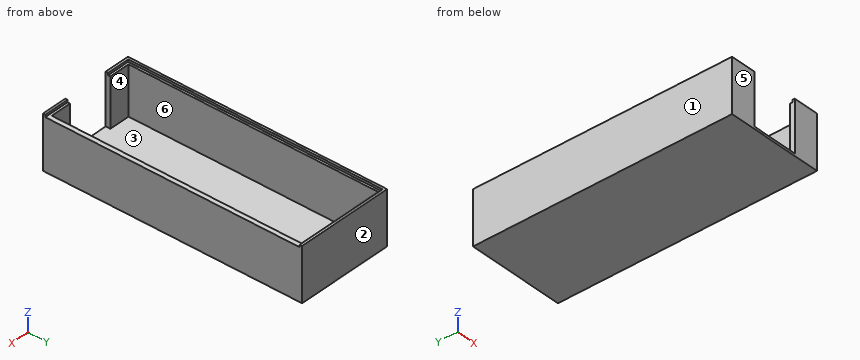
```python
from build123d import *

# Parameters (mm, degrees)
SKETCH_1_W          = 40
SKETCH_1_H          = 110
EXTRUDE_1_DEPTH     = 22
SHELL_1_T           = -1
SKETCH_17_W         = 20
SKETCH_17_H         = 21
CUT_EXTRUDE_3_DEPTH = 2
SKETCH_2_W          = 23
SKETCH_2_H          = 110
EXTRUDE_2_DEPTH     = 1
SKETCH_3_W          = 41
SKETCH_3_H          = 23
EXTRUDE_3_DEPTH     = 1
SKETCH_18_W         = 20
SKETCH_18_H         = 22
CUT_EXTRUDE_4_DEPTH = 2
SKETCH_5_W          = 41
SKETCH_5_H          = 23
EXTRUDE_4_DEPTH     = 1
SKETCH_9_W          = 22
SKETCH_9_H          = 112
EXTRUDE_5_DEPTH     = 1
SKETCH_10_W         = 1
SKETCH_10_H         = 1
EXTRUDE_6_DEPTH     = 1
SKETCH_11_W         = 1
SKETCH_11_H         = 1
EXTRUDE_7_DEPTH     = 1


with BuildPart() as part:
    # 스케치1 → 보스-돌출1 (new body)
    with BuildSketch(Plane.XY):
        with Locations((20, 55)):
            Rectangle(SKETCH_1_W, SKETCH_1_H)
    extrude(amount=EXTRUDE_1_DEPTH)

    # 쉘1
    shell_1_openings = [part.faces().sort_by_distance(p)[0] for p in [
        (20, 55, 22),
    ]]
    offset(amount=SHELL_1_T, openings=shell_1_openings, kind=Kind.INTERSECTION)

    # 스케치17 → 컷-돌출3 (cut, through all)
    with BuildSketch(Plane(origin=(0, 1, 0), x_dir=(1, 0, 0), z_dir=(0, 1, 0))):
        with Locations((20, -11.5)):
            Rectangle(SKETCH_17_W, SKETCH_17_H)
    extrude(amount=-CUT_EXTRUDE_3_DEPTH, mode=Mode.SUBTRACT)

    # 스케치2 → 보스-돌출2 (add)
    with BuildSketch(Plane.ZY):
        with Locations((11.5, 55)):
            Rectangle(SKETCH_2_W, SKETCH_2_H)
    extrude(amount=EXTRUDE_2_DEPTH)

    # 스케치3 → 보스-돌출3 (add)
    with BuildSketch(Plane.XZ):
        with Locations((19.5, 11.5)):
            Rectangle(SKETCH_3_W, SKETCH_3_H)
    extrude(amount=EXTRUDE_3_DEPTH)

    # 스케치18 → 컷-돌출4 (cut, through all)
    with BuildSketch(Plane(origin=(0, 0, 0), x_dir=(1, 0, 0), z_dir=(0, 1, 0))):
        with Locations((20, -12)):
            Rectangle(SKETCH_18_W, SKETCH_18_H)
    extrude(amount=-CUT_EXTRUDE_4_DEPTH, mode=Mode.SUBTRACT)

    # 스케치5 → 보스-돌출4 (add)
    with BuildSketch(Plane(origin=(0, 110, 0), x_dir=(1, 0, 0), z_dir=(0, 1, 0))):
        with Locations((19.5, -11.5)):
            Rectangle(SKETCH_5_W, SKETCH_5_H)
    extrude(amount=EXTRUDE_4_DEPTH)

    # 스케치9 → 보스-돌출5 (add)
    with BuildSketch(Plane(origin=(40, 0, 0), x_dir=(0, 0, -1), z_dir=(1, 0, 0))):
        with Locations((-11, 55)):
            Rectangle(SKETCH_9_W, SKETCH_9_H)
    extrude(amount=EXTRUDE_5_DEPTH)

    # 스케치10 → 보스-돌출6 (add)
    with BuildSketch(Plane.XY.offset(22)):
        with Locations((40.5, 110.5)):
            Rectangle(SKETCH_10_W, SKETCH_10_H)
    extrude(amount=EXTRUDE_6_DEPTH)

    # 스케치11 → 보스-돌출7 (add)
    with BuildSketch(Plane.XY.offset(22)):
        with Locations((40.5, -0.5)):
            Rectangle(SKETCH_11_W, SKETCH_11_H)
    extrude(amount=EXTRUDE_7_DEPTH)


solid = part.part
```
CAD build for the part. Positions are in the model's coordinates, mm. Face numbers are marked on the shaded views. A direction names the side the tool comes from. Coordinates: 2 decimals unless noted, no trailing zeros. Write each loop counter-clockwise with the first axis right and the second up, starting at its lowest first coordinate (ties: lowest second). Pieces come first, ordered by that corner, then holes. Notation, with made-up numbers: (-11.5, 10) -> (30.5, 10) arc R13 cw to (30.5, 18) -> close; hole circle Ø2 at (-39.5, -21). An arc over 180 degrees is marked (long way). Use CSV: the item, a comma, the result in double quotes. Start each with the question number.
Item 1: Two-plate mould, pull along Y, no slides. Class the marked faces 1, 2, 3 and 4: +Y half, -Y half, draft (parallel to the pull), parting line (faces both ways), or undercut.
Item 2: Tool access for the marked faces 5 and 6: list every direction of +Z, -Z, +X, -X, +Y, -Y with a clear straight run to the whole face (end or side of a thin tool).
Item 3: Band-saw the part on D-D, the plane x = 6. Write the cut outline in (y, z).
Item 4: Wall check: probe 1 along Y at (x, z) = (8, 1.75); probe 2 along X at (y, z) = (39, 3); probe 3 along Z at (x, y) = (2.5, 17). Give the ranges that are in metal, low to high.
Item 5: Drop flat-ended pins along their axis: P1, Ø6.5, axis at x = 20, z = 15, coming from the -Y side; P2, Ø12.5, axis at x = 11.5, y = 82.5, coming from the +Z side. Give the stop position or say it passes through.
Item 6: Band-saw the part on C-C, the plane y = 39. Write the cut outline in (x, z), plus the area to 3 significant figures.
Item 7: Band-saw the part on A-A, the plane z = 18.5. Write the cut outline in (x, y).
Item 8: Band-saw the part on B-B, the plane x = 25. Write the cut outline in (y, z), plus the area to 3 significant figures.
Response values:
1,face 1,"draft"
1,face 2,"+Y half"
1,face 3,"undercut"
1,face 4,"undercut"
2,face 5,"+Z, -Z, +X, -X, -Y"
2,face 6,"+Z"
3,outline,"(-1, 0) -> (111, 0) -> (111, 23) -> (110, 23) -> (110, 22) -> (109, 22) -> (109, 1) -> (1, 1) -> (1, 22) -> (0, 22) -> (0, 23) -> (-1, 23) -> close"
4,probe 1,"y = -1 to 1, 109 to 111"
4,probe 2,"x = -1 to 1, 39 to 41"
4,probe 3,"z = 0 to 1"
5,P1,"stops at y = 109"
5,P2,"stops at z = 1"
6,outline,"(-1, 0) -> (41, 0) -> (41, 22) -> (39, 22) -> (39, 1) -> (1, 1) -> (1, 22) -> (0, 22) -> (0, 23) -> (-1, 23) -> close"
6,area,"127 mm2"
7,outline,"(-1, -1) -> (10, -1) -> (10, 1) -> (1, 1) -> (1, 109) -> (39, 109) -> (39, 1) -> (30, 1) -> (30, -1) -> (41, -1) -> (41, 111) -> (-1, 111) -> close"
8,outline,"(-1, 0) -> (111, 0) -> (111, 23) -> (110, 23) -> (110, 22) -> (109, 22) -> (109, 1) -> (-1, 1) -> close"
8,area,"155 mm2"
